from build123d import *

# Parameters (mm, degrees)
SKETCH1_W           = 106.426
SKETCH1_H           = 63.5
BOSS_EXTRUDE1_DEPTH = 3.175
EDGE_FLANGE1_DEPTH  = 63.5


# Sheet-metal steps are written as plain solids
with BuildPart() as part:
    # Sketch1 → Boss-Extrude1 (new body)
    with BuildSketch(Plane(origin=(0, 0, 0), x_dir=(1, 0, 0), z_dir=(0, 1, 0))):
        with Locations((53.213, 31.75)):
            Rectangle(SKETCH1_W, SKETCH1_H)
    extrude(amount=BOSS_EXTRUDE1_DEPTH)

    # Edge-Flange1 section (across the edge) → Edge-Flange1 (add)
    with BuildSketch(Plane(origin=(107.188, 3.175, 0), x_dir=(-1, 0, 0), z_dir=(0, 0, -1))):
        with BuildLine():
            Line((-3.175, 0.762), (-3.175, 15.875))
            Line((-3.175, 15.875), (0, 15.875))
            Line((0, 15.875), (0, 0.762))
            ThreePointArc((0, 0.762), (0.223184633, 0.223184633), (0.762, 0))
            Line((0.762, 0), (0.762, -3.175))
            ThreePointArc((0.762, -3.175), (-2.021879398, -2.021879398), (-3.175, 0.762))
        make_face()
    extrude(amount=EDGE_FLANGE1_DEPTH)


solid = part.part
Source: CAD feature listing. Evaluate the final solid. Frame: model axes, mm. A direction names the side the tool comes from. Give positions to 0.01 mm unless a question says otherwise; leave off trailing zeros. Write each loop counter-clockwise with the first axis right and the second up, starting at its lowest first coordinate (ties: lowest second). Pieces come first, ordered by that corner, then holes. Notation, with made-up numbers: (-37.75, 47.25) -> (-2.75, 47.25) arc R38 ccw to (-2.75, 85.25) -> close; hole circle Ø6 at (5.25, -5). An arc over 180 degrees is marked (long way). Return JSON: item names as keys, results as strings. Group by question number.
1. Section A-A, the plane z = -43.5. Output: boundary loops of the cut face in (x, y) (3 decimals).
2. Section C-C, the plane y = 18. Output: boundary loops of the cut face in (x, z), then the cut area to 3 significant figures.
3. Section B-B, the plane x = 64.5. Output: boundary loops of the cut face in (y, z) (3 decimals).
4. Material intervals for line 1 (Y direction, x = 14, z = -9) (3 decimals); line 2 (X direction, y = 7.25, z = -28.5); line 3 (X direction, y = 3.5, z = -32.5), sorted ascending. Write a range as from..to.
5. Pin query (flat end, axial travel): pin 1 Ø10 at (y, z) = (8, -26) entering from -X; pin 2 Ø6 at (x, z) = (56, -20) entering from +Y (3 decimals); pin 3 Ø4.5 at (y, z) = (13.5, -42) entering from -X. Return the tip coordinate at first contact, or that it passes through.
6. Access query for faces 1 (the face through (107.188, 12, -31)), 2 (the face through (110.363, 11, -31)). Directions: +Z, -Z, +X, -X, +Y, -Y. A direction counts if a zero-diameter tool reaches every point of the face in a straight line with its end or side. Return the directions, or none.
Determined:
{
 "1": {"outline": "(0, 0) -> (106.426, 0) arc R3.937 ccw to (110.363, 3.937) -> (110.363, 19.05) -> (107.188, 19.05) -> (107.188, 3.937) arc R0.762 cw to (106.426, 3.175) -> (0, 3.175) -> close"},
 "2": {"outline": "(107.19, -63.5) -> (110.36, -63.5) -> (110.36, 0) -> (107.19, 0) -> close", "area": "202 mm2"},
 "3": {"outline": "(0, -63.5) -> (3.175, -63.5) -> (3.175, 0) -> (0, 0) -> close"},
 "4": {"line 1": "y = 0..3.175", "line 2": "x = 107.19..110.36", "line 3": "x = 107.05..110.34"},
 "5": {"pin 1": "stops at x = 0", "pin 2": "stops at y = 3.175", "pin 3": "stops at x = 107.19"},
 "6": {"face 1": "+Z, -Z, -X, +Y", "face 2": "+Z, -Z, +X, +Y, -Y"}
}
